Autodesk Inventor part; units mm, degrees
ref_plane "YZ Plane" through (0, 0, 0) normal (1, 0, 0) x (0, 1, 0)
ref_plane "XZ Plane" through (0, 0, 0) normal (0, 1, 0) x (-1, 0, 0)
ref_plane "XY Plane" through (0, 0, 0) normal (0, 0, 1) x (1, 0, 0)
sketch "Sketch1" plane through (0, 0, 0) normal (0, 1, 0) x (-1, 0, 0)
  line L0 (0, 0) -> (25, 0)
  line L1 (25, 0) -> (25, -25)
  line L2 (25, -25) -> (0, -25)
  line L3 (0, -25) -> (0, 0)
  circle A0 centre (12.5, -12.5) radius 11
  circle A1 centre (3.5, -3.5) radius 3.5
  circle A2 centre (3.5, -21.5) radius 3.5
  circle A3 centre (21.5, -21.5) radius 3.5
  circle A4 centre (21.5, -3.5) radius 3.5
  line L4 (25, -12.5) -> (0, -12.5) construction
  line L5 (12.5, -25) -> (12.5, 0) construction
  point P0 (6.9634, -2.995)
  point P1 (2.995, -6.9634)
  point P2 (18.0366, -2.995)
  point P3 (22.005, -6.9634)
  point P4 (6.9634, -22.005)
  point P5 (2.995, -18.0366)
  point P6 (22.005, -18.0366)
  point P7 (18.0366, -22.005)
  point P8 (0, -3.5)
  point P9 (3.5, 0)
  point P10 (25, -3.5)
  point P11 (21.5, 0)
  point P12 (0, -21.5)
  point P13 (3.5, -25)
  point P14 (21.5, -25)
  point P15 (25, -21.5)
  dimension "cellRadius" = 22
  dimension "catcherRadius" = 7
  dimension "d27" = 7
  dimension "d28" = 7
  dimension "d29" = 7
  dimension "d36" = 25
  dimension "d37" = 25
extrude "thickness" add sketch "Sketch1" along normal blind 6 contours L0 A1 L3 | L0 A4 A0 A1 | A1 A0 | A1 A0 A2 L3 | L0 L1 A4 | A4 A0 | A2 L2 L3 | A2 A0 | L1 A3 A0 A4 | A2 A0 A3 L2 | A3 A0 | L1 L2 A3 picked at (3.6063, -3.4216) picked at (21.3937, -3.4216) picked at (3.4216, -21.3937) picked at (21.3937, -21.5784)
extrude "catcher" add sketch "Sketch1" along normal blind 1 contours L0 A1 L3 | A1 A0 | L0 L1 A4 | A4 A0 | A1 A0 | A2 L2 L3 | A2 A0 | A0 A4 | A2 A0 | A3 A0 | L1 L2 A3 | A0 A3
equation "\"d27\" = catcherRadius"
equation "\"d28\" = catcherRadius"
equation "\"d29\" = catcherRadius"
equation "\"d36\" = width"
equation "\"d37\" = width"
equation "\"catcherHeight\" = 0.166667 * spacerHeight"
properties part number "spacers_base"
CAD build for the part. Positions are in the model's coordinates, mm. A direction names the side the tool comes from. Coordinates: 2 decimals unless noted, no trailing zeros. Loops run counter-clockwise (first coordinate to the right, second up) from the corner with the lowest first, then second, coordinate; pieces in that order, holes last. Notation, with made-up numbers: (-3.5, -10) -> (15.5, -10) arc R24 ccw to (15.5, 20) -> close; hole circle Ø8 at (-28.5, 76.25). An arc over 180 degrees is marked (long way). One line per item, written item: value.
1. Slice it at D-D on z = -20.5. Write the cut outline in (x, y).
Answers:
outline: (-25, 0) -> (-18.15, 0) -> (-18.15, 1) -> (-20.05, 1) -> (-20.05, 6) -> (-25, 6) -> close; (-6.85, 0) -> (0, 0) -> (0, 6) -> (-4.95, 6) -> (-4.95, 1) -> (-6.85, 1) -> close
2. Slice it at C-C on y = 3.9. Write the cut outline in (x, z), and give its area (3 significant figures).
Answers:
outline: (-25, -25) -> (0, -25) -> (0, 0) -> (-25, 0) -> close; hole circle Ø22 at (-12.5, -12.5)
area: 245 mm^2
3. Flat gauge pin, fed straight in: P1, Ø1.2, axis at x = -19.5, z = -5.5, coming from the +Y side. Where does the tip first touch, or does it go through?
Answers:
P1: stops at y = 1
4. Slice it at A-A on x = -12.5. Write the cut outline in (y, z), and give its area (3 significant figures).
Answers:
outline: (0, -25) -> (6, -25) -> (6, -23.5) -> (0, -23.5) -> close; (0, -1.5) -> (6, -1.5) -> (6, 0) -> (0, 0) -> close
area: 18.0 mm^2
5. Pull direction X, two halves, no side cores. Call faces 1 (the face through (-5, 1, -5)), 2 (the face through (-25, 3, -12)), 3 (the face through (-4, 0, -6.8)): pulls with the +X half, pulls with the -X half, needs draft (parallel to the pull), parting line crosses it, or undercut.
Answers:
face 1: undercut
face 2: pulls with the -X half
face 3: needs draft
6. Which spindle directions (+Z, -Z, +X, -X, +Y, -Y) get a long thin tool onto all of the face, cutting with end or side? Do faces 4 (the face through (-20, 1, -5)), 5 (the face through (-1, 6, -12)), 6 (the face through (-6.01, 0.49, -5.94)). Say none if no direction does.
Answers:
face 4: +Y
face 5: +Z, -Z, +X, -X, +Y
face 6: +Y, -Y
7. Slice it at B-B on z = -12.5. Write the cut outline in (x, y), and give its area (3 significant figures).
Answers:
outline: (-25, 0) -> (-23.5, 0) -> (-23.5, 6) -> (-25, 6) -> close; (-1.5, 0) -> (0, 0) -> (0, 6) -> (-1.5, 6) -> close
area: 18.0 mm^2
8. Drill centre lines: line 1 (X direction, y = 4, z = -12.5); line 2 (X direction, y = 3.4, z = -17.25). Where is each one in solid material? Low to high. Write a range as [from, to].
Answers:
line 1: x = [-25, -23.5], [-1.5, 0]
line 2: x = [-25, -22.42], [-2.58, 0]
